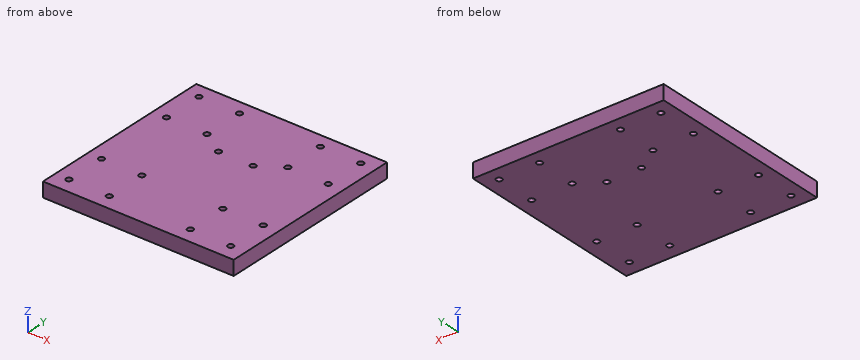
from build123d import *

# Parameters (mm, degrees)
CROQUIS1_W              = 165
CROQUIS1_H              = 165
CROQUIS1_R              = 2.5
SALIENTE_EXTRUIR1_DEPTH = 12.7
CORTAR_EXTRUIR1_START   = -12.7
CROQUIS2_R              = 2.5
CORTAR_EXTRUIR1_DEPTH   = 12.7


with BuildPart() as part:
    # Croquis1 → Saliente-Extruir1 (new body)
    with BuildSketch(Plane.XY):
        Rectangle(CROQUIS1_W, CROQUIS1_H)
        with Locations((-70.5, 70.5)):
            Circle(CROQUIS1_R, mode=Mode.SUBTRACT)
        with Locations((-35.5, 70.5)):
            Circle(CROQUIS1_R, mode=Mode.SUBTRACT)
        with Locations((-35.5, 35.5)):
            Circle(CROQUIS1_R, mode=Mode.SUBTRACT)
        with Locations((-70.5, 35.5)):
            Circle(CROQUIS1_R, mode=Mode.SUBTRACT)
        with Locations((34.5, 70.5)):
            Circle(CROQUIS1_R, mode=Mode.SUBTRACT)
        with Locations((69.5, 70.5)):
            Circle(CROQUIS1_R, mode=Mode.SUBTRACT)
        with Locations((69.5, 35.5)):
            Circle(CROQUIS1_R, mode=Mode.SUBTRACT)
        with Locations((34.5, 35.5)):
            Circle(CROQUIS1_R, mode=Mode.SUBTRACT)
        with Locations((34.5, -34.5)):
            Circle(CROQUIS1_R, mode=Mode.SUBTRACT)
        with Locations((69.5, -34.5)):
            Circle(CROQUIS1_R, mode=Mode.SUBTRACT)
        with Locations((69.5, -69.5)):
            Circle(CROQUIS1_R, mode=Mode.SUBTRACT)
        with Locations((34.5, -69.5)):
            Circle(CROQUIS1_R, mode=Mode.SUBTRACT)
        with Locations((-70.5, -34.5)):
            Circle(CROQUIS1_R, mode=Mode.SUBTRACT)
        with Locations((-35.5, -34.5)):
            Circle(CROQUIS1_R, mode=Mode.SUBTRACT)
        with Locations((-35.5, -69.5)):
            Circle(CROQUIS1_R, mode=Mode.SUBTRACT)
        with Locations((-70.5, -69.5)):
            Circle(CROQUIS1_R, mode=Mode.SUBTRACT)
    extrude(amount=SALIENTE_EXTRUIR1_DEPTH)

    # Croquis2 → Cortar-Extruir1 (cut)
    with BuildSketch(Plane.XY.offset(12.7).offset(CORTAR_EXTRUIR1_START)):
        with Locations((-15, 22.390106488)):
            Circle(CROQUIS2_R)
        with Locations((15, 22.390106488)):
            Circle(CROQUIS2_R)
        with Locations((69.5, -69.5)):
            Circle(CROQUIS2_R)
        with Locations((69.5, -34.5)):
            Circle(CROQUIS2_R)
        with Locations((34.5, -69.5)):
            Circle(CROQUIS2_R)
        with Locations((34.5, -34.5)):
            Circle(CROQUIS2_R)
        with Locations((-35.5, -69.5)):
            Circle(CROQUIS2_R)
        with Locations((-70.5, -69.5)):
            Circle(CROQUIS2_R)
        with Locations((-35.5, -34.5)):
            Circle(CROQUIS2_R)
        with Locations((-70.5, -34.5)):
            Circle(CROQUIS2_R)
        with Locations((69.5, 35.5)):
            Circle(CROQUIS2_R)
        with Locations((34.5, 35.5)):
            Circle(CROQUIS2_R)
        with Locations((69.5, 70.5)):
            Circle(CROQUIS2_R)
        with Locations((34.5, 70.5)):
            Circle(CROQUIS2_R)
        with Locations((-35.5, 35.5)):
            Circle(CROQUIS2_R)
        with Locations((-70.5, 35.5)):
            Circle(CROQUIS2_R)
        with Locations((-35.5, 70.5)):
            Circle(CROQUIS2_R)
        with Locations((-70.5, 70.5)):
            Circle(CROQUIS2_R)
    extrude(amount=CORTAR_EXTRUIR1_DEPTH, mode=Mode.SUBTRACT)


solid = part.part
Geometry: final body of the model. Coordinates: model frame, mm. Round coordinates to 2 decimals unless told otherwise and drop trailing zeros. Loops run counter-clockwise (first coordinate to the right, second up) from the corner with the lowest first, then second, coordinate; pieces in that order, holes last. Notation, with made-up numbers: M -39.5,-15 L -14.5,-15 A11 cw -14.5,-8 Z; hole C 28.25,-34.75 d5. An arc over 180 degrees is marked long. Put each result on its own line as item: value. Start each with the question number.
(1) Section query B-B (x = -70.5). Return loops of the section in (y, z), then the cut area to 3 significant figures.
(2) Material intervals for line 1 along Y through (x, z) = (-70.5, 3.75); line 2 along X through (y, z) = (-34, 1), sorted ascending. Write a range as [from, to].
(3) Section query C-C (x = -15). Return loops of the section in (y, z), then the cut area to 3 significant figures.
(4) Section query A-A (y = -34.5). Return loops of the section in (x, z).
Findings below:
1. outline: M -82.5,0 L -72,0 L -72,12.7 L -82.5,12.7 Z; M -67,0 L -37,0 L -37,12.7 L -67,12.7 Z; M -32,0 L 33,0 L 33,12.7 L -32,12.7 Z; M 38,0 L 68,0 L 68,12.7 L 38,12.7 Z; M 73,0 L 82.5,0 L 82.5,12.7 L 73,12.7 Z
1. area: 1,840 mm2
2. line 1: y = [-82.5, -72], [-67, -37], [-32, 33], [38, 68], [73, 82.5]
2. line 2: x = [-82.5, -72.95], [-68.05, -37.95], [-33.05, 32.05], [36.95, 67.05], [71.95, 82.5]
3. outline: M -82.5,0 L 19.89,0 L 19.89,12.7 L -82.5,12.7 Z; M 24.89,0 L 82.5,0 L 82.5,12.7 L 24.89,12.7 Z
3. area: 2,030 mm2
4. outline: M -82.5,0 L -73,0 L -73,12.7 L -82.5,12.7 Z; M -68,0 L -38,0 L -38,12.7 L -68,12.7 Z; M -33,0 L 32,0 L 32,12.7 L -33,12.7 Z; M 37,0 L 67,0 L 67,12.7 L 37,12.7 Z; M 72,0 L 82.5,0 L 82.5,12.7 L 72,12.7 Z
